Here's how the part is built. I have some questions about the finished solid (model axes, mm). A direction names the side the tool comes from. Round coordinates to 2 decimals unless told otherwise and drop trailing zeros. Order: outer loops, then holes, each group sorted by start corner. A loop starts at its lowest first (then second) coordinate and runs counter-clockwise, first axis right, second up. Notation, with made-up numbers: (24.5, 72.5) -> (57.5, 72.5) arc R30 cw to (57.5, 106.5) -> close; hole circle Ø3 at (63, 64). An arc over 180 degrees is marked (long way). Answer in a Markdown table with one row per item.
```python
from build123d import *

# Parameters (mm, degrees)
SKETCH1_W           = 136
SKETCH1_H           = 66
BOSS_EXTRUDE1_DEPTH = 48
CUT_EXTRUDE1_START  = 8
SKETCH2_W           = 37.33
SKETCH2_H           = 54
SKETCH2_W_2         = 37.34
CUT_EXTRUDE1_DEPTH  = 48
FILLET1_R           = 20


with BuildPart() as part:
    # Sketch1 → Boss-Extrude1 (new body)
    with BuildSketch(Plane(origin=(0, 0, 0), x_dir=(1, 0, 0), z_dir=(0, 1, 0))):
        Rectangle(SKETCH1_W, SKETCH1_H)
    extrude(amount=BOSS_EXTRUDE1_DEPTH)

    # Sketch2 → Cut-Extrude1 (cut)
    with BuildSketch(Plane(origin=(0, 48, 0), x_dir=(1, 0, 0), z_dir=(0, 1, 0)).offset(CUT_EXTRUDE1_START)):
        with Locations((-43.335, 0)):
            Rectangle(SKETCH2_W, SKETCH2_H)
        Rectangle(SKETCH2_W_2, SKETCH2_H)
        with Locations((43.335, 0)):
            Rectangle(SKETCH2_W, SKETCH2_H)
    extrude(amount=-CUT_EXTRUDE1_DEPTH, mode=Mode.SUBTRACT)

    # Fillet1
    fillet1_edges = [part.edges().sort_by_distance(p)[0] for p in [
        (-43.335, 8, -27),
        (-43.335, 8, 27),
        (0, 8, -27),
        (0, 8, 27),
        (43.335, 8, -27),
        (43.335, 8, 27),
    ]]
    fillet(fillet1_edges, radius=FILLET1_R)


solid = part.part
```
1. Suppose I cut it at B-B on x = -7. Write out the boundary of the cut face in (y, z), then the cut area to 3 significant figures.
Numbers:
| item | result |
|---|---|
| outline | (0, -33) -> (48, -33) -> (48, -27) -> (28, -27) arc R20 cw to (8, -7) -> (8, 7) arc R20 cw to (28, 27) -> (48, 27) -> (48, 33) -> (0, 33) -> close |
| area | 1,180 mm2 |
2. We'd pull the mould along X, two halves only. Please class faces 1 (the face through (-1, 24, 33)), 2 (the face through (68, 24, 0)), 3 (the face through (0.261, 14.014, -21.297)): released by +X, released by -X, zero draft, split by the parting line, or undercut.
Numbers:
| item | result |
|---|---|
| face 1 | zero draft |
| face 2 | released by +X |
| face 3 | undercut |
3. For pin 1 Ø11 at (x, z) = (39.5, 2) entering from +Y, with a flat end and sliding along its axis, tell me the tip position at first contact or that it passes through.
Numbers:
| item | result |
|---|---|
| pin 1 | stops at y = 8.01 |
4. Please list where these lines run through material, in increasing order: line 1 along X through (y, z) = (27.5, 13.5); line 2 along Z through (x, y) = (54, 40); line 3 along Y through (x, z) = (-6, -7).
Numbers:
| item | result |
|---|---|
| line 1 | x = -68 to -62, -24.67 to -18.67, 18.67 to 24.67, 62 to 68 |
| line 2 | z = -33 to -27, 27 to 33 |
| line 3 | y = 0 to 8 |
5. Suppose I cut it at D-D on y = 15. Write out the boundary of the cut face in (x, z), then the cut area to 3 significant figures.
Numbers:
| item | result |
|---|---|
| outline | (-68, -33) -> (68, -33) -> (68, 33) -> (-68, 33) -> close; hole (-62, -22.2) -> (-24.67, -22.2) -> (-24.67, 22.2) -> (-62, 22.2) -> close; hole (-18.67, -22.2) -> (18.67, -22.2) -> (18.67, 22.2) -> (-18.67, 22.2) -> close; hole (24.67, -22.2) -> (62, -22.2) -> (62, 22.2) -> (24.67, 22.2) -> close |
| area | 4,000 mm2 |
6. Suppose I cut it at A-A on y = 37. Write out the boundary of the cut face in (x, z).
Numbers:
| item | result |
|---|---|
| outline | (-68, -33) -> (68, -33) -> (68, 33) -> (-68, 33) -> close; hole (-62, -27) -> (-24.67, -27) -> (-24.67, 27) -> (-62, 27) -> close; hole (-18.67, -27) -> (18.67, -27) -> (18.67, 27) -> (-18.67, 27) -> close; hole (24.67, -27) -> (62, -27) -> (62, 27) -> (24.67, 27) -> close |
7. For faces 4 (the face through (20, 48, 0)), 5 (the face through (43.596, 14.014, 21.297)), which set-ups out of +Z, -Z, +X, -X, +Y, -Y let a thin tool reach every point of the face, with its end or its side?
Numbers:
| item | result |
|---|---|
| face 4 | +Z, -Z, +X, -X, +Y |
| face 5 | +Y |
8. Suppose I cut it at C-C on z = -19. Write out the boundary of the cut face in (x, y), then the cut area to 3 significant figures.
Numbers:
| item | result |
|---|---|
| outline | (-68, 0) -> (68, 0) -> (68, 48) -> (62, 48) -> (62, 12) -> (24.67, 12) -> (24.67, 48) -> (18.67, 48) -> (18.67, 12) -> (-18.67, 12) -> (-18.67, 48) -> (-24.67, 48) -> (-24.67, 12) -> (-62, 12) -> (-62, 48) -> (-68, 48) -> close |
| area | 2,500 mm2 |
